from build123d import *

# Parameters (mm, degrees)
SKETCH1_W           = 17.78
SKETCH1_H           = 46.228
BOSS_EXTRUDE1_DEPTH = 4.9022
SKETCH2_R           = 1.9939
SKETCH2_R_2         = 2.032
BOSS_EXTRUDE2_DEPTH = 11.8618
SKETCH3_R           = 1.6383
CUT_EXTRUDE1_DEPTH  = 17.764


with BuildPart() as part:
    # Sketch1 → Boss-Extrude1 (new body)
    with BuildSketch(Plane(origin=(0, 0, 0), x_dir=(1, 0, 0), z_dir=(0, 1, 0))):
        with Locations((-7.973944862, -11.637942607)):
            Rectangle(SKETCH1_W, SKETCH1_H)
    extrude(amount=BOSS_EXTRUDE1_DEPTH)

    # Sketch2 → Boss-Extrude2 (add)
    with BuildSketch(Plane.XZ):
        with Locations((-14.577944862, 32.465942607)):
            Circle(SKETCH2_R)
        with Locations((-1.369944862, 32.465942607)):
            Circle(SKETCH2_R_2)
        with Locations((-1.369944862, -9.190057393)):
            Circle(SKETCH2_R_2)
        with Locations((-14.577944862, -9.190057393)):
            Circle(SKETCH2_R_2)
    extrude(amount=BOSS_EXTRUDE2_DEPTH)

    # Sketch3 → Cut-Extrude1 (cut, through all)
    with BuildSketch(Plane.XZ.offset(11.8618)):
        with Locations((-14.577944862, 32.465942607)):
            Circle(SKETCH3_R)
        with Locations((-14.577944862, -9.190057393)):
            Circle(SKETCH3_R)
        with Locations((-1.369944862, -9.190057393)):
            Circle(SKETCH3_R)
        with Locations((-1.369944862, 32.465942607)):
            Circle(SKETCH3_R)
    extrude(amount=-CUT_EXTRUDE1_DEPTH, mode=Mode.SUBTRACT)


solid = part.part
For this review, take the finished solid that the model builds, in its own axes (mm). A direction names the side the tool comes from. Round coordinates to 2 decimals unless told otherwise and drop trailing zeros. Loops run counter-clockwise (first coordinate to the right, second up) from the corner with the lowest first, then second, coordinate; pieces in that order, holes last. Notation, with made-up numbers: (48.5, 59.5) - (97.5, 59.5) arc R28 ccw to (97.5, 78.5) - close; hole circle Ø1 at (52, 9). An arc over 180 degrees is marked (long way). Use one line per item in the form item = value.
Item 1: Tool access review of faces 1 (the cylindrical face through (-12.7, -5.85, -9.97)), 2 (the flat face through (-16, -11.862, -8)): name each direction out of +Z, -Z, +X, -X, +Y, -Y from which nothing blocks a thin tool from reaching the whole face with its end or side.
Answers:
face_1 = -Y
face_2 = +Z, -Z, +X, -X, -Y
Item 2: Consider section A-A on y = -3.5. Write out the cut boundary in (x, z).
Answers:
outline = circle Ø4.06 at (-14.58, -9.19); circle Ø3.99 at (-14.58, 32.47); circle Ø4.06 at (-1.37, -9.19); circle Ø4.06 at (-1.37, 32.47); hole circle Ø3.28 at (-14.58, -9.19); hole circle Ø3.28 at (-14.58, 32.47); hole circle Ø3.28 at (-1.37, -9.19); hole circle Ø3.28 at (-1.37, 32.47)
Item 3: Mouldability with a two-part tool opening along X and no side actions: class faces 3 (the flat face through (-8, 2, 34.752)), 4 (the flat face through (0.916, 2, 12)), 5 (the cylindrical face through (-1.63, -5.85, 34.48)) as +X half, -X half, draft (parallel to the pull), parting line (faces both ways), or undercut.
Answers:
face_3 = draft
face_4 = +X half
face_5 = undercut
Item 4: Clearance check with a flat-ended pin moving along its axis: P1, Ø3, axis at x = -13, z = 13.5, coming from the -Y side. State where the tip first meets the part, or that it passes through.
Answers:
P1 = 0
Item 5: Consider section B-B on x = -0.25. Write out the cut boundary in (y, z), then the cut area to 3 significant figures.
Answers:
outline = (-11.86, -10.89) - (0, -10.89) - (0, -11.48) - (4.9, -11.48) - (4.9, -10.39) - (-11.86, -10.39) - close; (-11.86, -7.99) - (4.9, -7.99) - (4.9, 31.27) - (-11.86, 31.27) - (-11.86, 30.77) - (0, 30.77) - (0, -7.49) - (-11.86, -7.49) - close; (-11.86, 33.66) - (4.9, 33.66) - (4.9, 34.75) - (0, 34.75) - (0, 34.16) - (-11.86, 34.16) - close
area = 227 mm^2
Item 6: Consider section D-D on y = 2.5. Write out the cut boundary in (x, z), then the cut area to 3 significant figures.
Answers:
outline = (-16.86, -11.48) - (0.92, -11.48) - (0.92, 34.75) - (-16.86, 34.75) - close; hole circle Ø3.28 at (-14.58, -9.19); hole circle Ø3.28 at (-14.58, 32.47); hole circle Ø3.28 at (-1.37, -9.19); hole circle Ø3.28 at (-1.37, 32.47)
area = 788 mm^2
Item 7: Consider section C-C on z = 25. Write out the cut boundary in (x, y), then the cut area to 3 significant figures.
Answers:
outline = (-16.86, 0) - (0.92, 0) - (0.92, 4.9) - (-16.86, 4.9) - close
area = 87.2 mm^2
Item 8: For line 1 (Z direction, x = -14.75, y = -6); line 2 (Z direction, x = -1, y = -9.25); line 3 (Y direction, x = -14, z = 7.5), list the stretches that pass through material, from the lowest coordinate up.
Answers:
line_1 = -11.21 to -10.82, -7.56 to -7.17, 30.48 to 30.84, 34.1 to 34.45
line_2 = -11.19 to -10.79, -7.59 to -7.19, 30.47 to 30.87, 34.06 to 34.46
line_3 = 0 to 4.9
